from build123d import *

# Parameters (mm, degrees)
BOSS_EXTRUDE1_DEPTH    = 12.446
CUT_EXTRUDE1_DEPTH     = 145.222130465
F_10_CLEARANCE_HOLE1_D = 5.1054
CUT_EXTRUDE2_DEPTH     = 145.222130465


with BuildPart() as part:
    # Sketch1 → Boss-Extrude1 (new body)
    with BuildSketch(Plane.XY):
        Polygon((0, 0), (0, 25.4), (3.2385, 25.4), (3.2385, 101.6), (22.1615, 101.6), (22.1615, 25.4), (25.4, 25.4), (25.4, 22.1615), (101.6, 22.1615), (101.6, 3.2385), (25.4, 3.2385), (25.4, 0), align=None)
    extrude(amount=BOSS_EXTRUDE1_DEPTH)

    # Sketch2 → Cut-Extrude1 (cut, through all)
    with BuildSketch(Plane.XY.offset(12.446)):
        with BuildLine():
            Line((6.35, 25.4), (0, 25.4))
            Line((0, 25.4), (0, 0))
            Line((0, 0), (19.05, 0))
            Line((19.05, 0), (19.05, 12.7))
            ThreePointArc((19.05, 12.7), (15.330256121, 21.680256121), (6.35, 25.4))
        make_face()
    extrude(amount=-CUT_EXTRUDE1_DEPTH, mode=Mode.SUBTRACT)

    # #10 Clearance Hole1 (through all)
    with Locations(Plane.XY.offset(12.446)):
        with Locations((88.9, 12.7), (8.001, 88.9), (8.001, 63.5), (8.001, 38.1), (38.1, 12.7), (63.5, 12.7)):
            Hole(F_10_CLEARANCE_HOLE1_D / 2)

    # Sketch5 → Cut-Extrude2 (cut, through all)
    with BuildSketch(Plane.XY.offset(12.446)):
        Polygon((13.081, 85.967060633), (13.081, 91.832939367), (8.001, 94.765878735), (2.921, 91.832939367), (2.921, 85.967060633), (8.001, 83.034121265), align=None)
        Polygon((13.081, 60.567060633), (13.081, 66.432939367), (8.001, 69.365878735), (2.921, 66.432939367), (2.921, 60.567060633), (8.001, 57.634121265), align=None)
        Polygon((13.081, 35.167060633), (13.081, 41.032939367), (8.001, 43.965878735), (2.921, 41.032939367), (2.921, 35.167060633), (8.001, 32.234121265), align=None)
        Polygon((41.032939367, 7.62), (43.965878735, 12.7), (41.032939367, 17.78), (35.167060633, 17.78), (32.234121265, 12.7), (35.167060633, 7.62), align=None)
        Polygon((66.432939367, 7.62), (69.365878735, 12.7), (66.432939367, 17.78), (60.567060633, 17.78), (57.634121265, 12.7), (60.567060633, 7.62), align=None)
        Polygon((91.832939367, 7.62), (94.765878735, 12.7), (91.832939367, 17.78), (85.967060633, 17.78), (83.034121265, 12.7), (85.967060633, 7.62), align=None)
    extrude(amount=-CUT_EXTRUDE2_DEPTH, mode=Mode.SUBTRACT)


solid = part.part
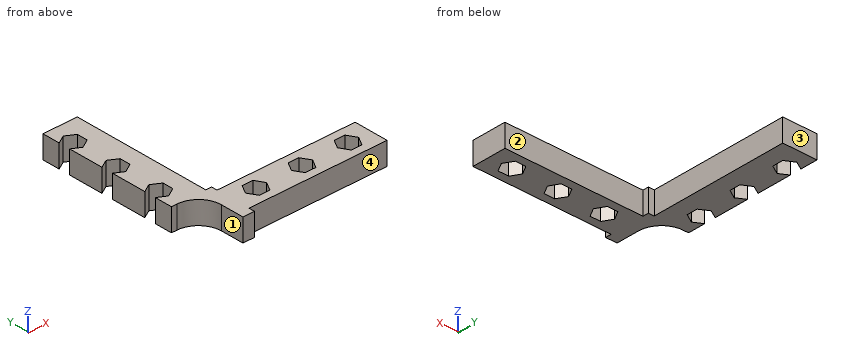
The listing builds one solid part. Answer for the finished solid, in the listing's coordinates (mm). Face numbers are marked on the shaded views. A direction names the side the tool comes from. Give positions to 0.01 mm unless a question says otherwise; leave off trailing zeros. Loops run counter-clockwise (first coordinate to the right, second up) from the corner with the lowest first, then second, coordinate; pieces in that order, holes last.
Item 1: A cutting plane is placed at D-D (y = 19.5). Give the vertices of the cut face in (x, z).
Derived:
outline: (17.08, 0) - (101.6, 0) - (101.6, 12.45) - (17.08, 12.45) - close
Item 2: Each of these flat-tipped pins is pushed along its axis until it touches: pin 1 Ø2 at (x, z) = (31, 4.5) entering from -Y; pin 2 Ø3.5 at (y, z) = (82.5, 6) entering from +X; pin 3 Ø1 at (y, z) = (1, 9.5) entering from +X. Where does it stop, or does it pass through?
Derived:
pin 1: stops at y = 3.24
pin 2: stops at x = 22.16
pin 3: stops at x = 25.4
Item 3: A cutting plane is placed at B-B (z = 10). Give the number of separate pieces and of enclosed holes in the cut face, then the cut area to 3 significant figures.
Derived:
separate pieces: 1
enclosed holes: 3
area: 2,550 mm2
Item 4: Find the intervals of material crossed by line 1 along Y through (x, z) = (91.5, 1.25); line 2 along Y through (x, z) = (7, 2); line 3 along Y through (x, z) = (24, 11.5), in increasing order.
Derived:
line 1: y = 3.24 to 7.62, 17.78 to 22.16
line 2: y = 25.38 to 32.81, 43.39 to 58.21, 68.79 to 83.61, 94.19 to 101.6
line 3: y = 0 to 25.4
Item 5: A cutting plane is placed at A-A (x = 37). Give the vertices of the cut face in (y, z).
Derived:
outline: (3.24, 0) - (7.62, 0) - (7.62, 12.45) - (3.24, 12.45) - close; (17.78, 0) - (22.16, 0) - (22.16, 12.45) - (17.78, 12.45) - close
Item 6: A cutting plane is placed at C-C (y = 80). Give the vertices of the cut face in (x, z).
Derived:
outline: (3.24, 0) - (22.16, 0) - (22.16, 12.45) - (3.24, 12.45) - close
Item 7: A tool of negligible diameter and unlimited length cuts with its end or side. For the marked faces 1, 2, 3 and 4, from which of +Z, -Z, +X, -X, +Y, -Y can it reach the whole face along a straight path? Write none if from no direction.
Derived:
face 1: +Z, -Z, -X, -Y
face 2: +Z, -Z, +X, +Y
face 3: +Z, -Z, +X, -X, +Y
face 4: +Z, -Z, +X, -Y
